CAD build for the part. Positions are in the model's coordinates, mm. Face numbers are marked on the shaded views. A direction names the side the tool comes from. Give positions to 0.01 mm unless a question says otherwise; leave off trailing zeros. Loops run counter-clockwise (first coordinate to the right, second up) from the corner with the lowest first, then second, coordinate; pieces in that order, holes last. Notation, with made-up numbers: (86, 31) -> (135, 31) arc R28 ccw to (135, 59) -> close; hole circle Ø3 at (79.25, 45.25). An arc over 180 degrees is marked (long way). Use one line per item in the form item = value.
```python
from build123d import *

# Parameters (mm, degrees)
F2_W     = 3
F2_H     = 3
F3_DEPTH = 9.201
F4_R     = 0.7
F5_DEPTH = 11.301


with BuildPart() as f1:
    # F0 (on Front) → F1 (revolve)
    with BuildSketch(Plane.XZ):
        Polygon((9.2, 8.05), (0, 8.05), (0.8, 6.6643593539), (0.8, 2.4), (9.4, 2.4), (10.3, 1.5), (14.8, 1.5), (14.8, 1.7), (27.8, 1.7), (27.8, 1.5), (33.8, 1.5), (33.8, 2.5), (33.2, 2.5), (33.2, 2.3), (32.5, 2.3), (32.5, 2.7), (12.1, 2.7), (12.1, 2.6), (11.3, 2.6), (11.3, 10), (9.2, 10), align=None)
    revolve(axis=Axis((16.7398190946, 0, 0), (1, 0, 0)))

    # F2 (on face) → F3 (cut, through all)
    with BuildSketch(Plane(origin=(9.2, 0, 0), x_dir=(0, -1, 0), z_dir=(-1, 0, 0))):
        with BuildLine():
            Line((1.5, 1.5), (1.5, 7.909013845))
            ThreePointArc((1.5, 7.909013845), (0, 8.05), (-1.5, 7.909013845))
            Line((-1.5, 7.909013845), (-1.5, 1.5))
            Line((-1.5, 1.5), (1.5, 1.5))
        make_face()
        with BuildLine():
            Line((1.5, 7.909013845), (1.5, 9.8868599666))
            ThreePointArc((1.5, 9.8868599666), (0, 10), (-1.5, 9.8868599666))
            Line((-1.5, 9.8868599666), (-1.5, 7.909013845))
            ThreePointArc((-1.5, 7.909013845), (0, 8.05), (1.5, 7.909013845))
        make_face()
        with BuildLine():
            Line((-1.5, -1.5), (-1.5, 1.5))
            Line((-1.5, 1.5), (-7.909013845, 1.5))
            ThreePointArc((-7.909013845, 1.5), (-8.05, 0), (-7.909013845, -1.5))
            Line((-7.909013845, -1.5), (-1.5, -1.5))
        make_face()
        with BuildLine():
            Line((-7.909013845, 1.5), (-9.8868599666, 1.5))
            ThreePointArc((-9.8868599666, 1.5), (-10, 0), (-9.8868599666, -1.5))
            Line((-9.8868599666, -1.5), (-7.909013845, -1.5))
            ThreePointArc((-7.909013845, -1.5), (-8.05, 0), (-7.909013845, 1.5))
        make_face()
        Rectangle(F2_W, F2_H)
        with BuildLine():
            ThreePointArc((8.05, 0), (8.0146759589, 0.7533055648), (7.909013845, 1.5))
            Line((7.909013845, 1.5), (1.5, 1.5))
            Line((1.5, 1.5), (1.5, -1.5))
            Line((1.5, -1.5), (7.909013845, -1.5))
            ThreePointArc((7.909013845, -1.5), (8.0146759589, -0.7533055648), (8.05, 0))
        make_face()
        with BuildLine():
            ThreePointArc((9.8868599666, -1.5), (9.971674876, -0.7521304187), (10, 0))
            ThreePointArc((10, 0), (9.971674876, 0.7521304187), (9.8868599666, 1.5))
            Line((9.8868599666, 1.5), (7.909013845, 1.5))
            ThreePointArc((7.909013845, 1.5), (8.0146759589, 0.7533055648), (8.05, 0))
            ThreePointArc((8.05, 0), (8.0146759589, -0.7533055648), (7.909013845, -1.5))
            Line((7.909013845, -1.5), (9.8868599666, -1.5))
        make_face()
        with BuildLine():
            ThreePointArc((-1.5, -7.909013845), (0, -8.05), (1.5, -7.909013845))
            Line((1.5, -7.909013845), (1.5, -1.5))
            Line((1.5, -1.5), (-1.5, -1.5))
            Line((-1.5, -1.5), (-1.5, -7.909013845))
        make_face()
        with BuildLine():
            ThreePointArc((-1.5, -9.8868599666), (0, -10), (1.5, -9.8868599666))
            Line((1.5, -9.8868599666), (1.5, -7.909013845))
            ThreePointArc((1.5, -7.909013845), (0, -8.05), (-1.5, -7.909013845))
            Line((-1.5, -7.909013845), (-1.5, -9.8868599666))
        make_face()
    extrude(amount=F3_DEPTH, mode=Mode.SUBTRACT)

    # F4 (on face) → F5 (cut, through all)
    with BuildSketch(Plane.YZ.offset(11.3)):
        with BuildLine():
            Line((-5.0204581464, 6.4346717088), (-6.3285168585, 7.7427304209))
            ThreePointArc((-6.3285168585, 7.7427304209), (-7.0710678119, 7.0710678119), (-7.7427304209, 6.3285168585))
            Line((-7.7427304209, 6.3285168585), (-6.4346717088, 5.0204581464))
            Line((-6.4346717088, 5.0204581464), (-5.0204581464, 6.4346717088))
        make_face()
        with Locations((0, 3.5)):
            Circle(F4_R)
        with Locations((0, -3.5)):
            Circle(F4_R)
    extrude(amount=-F5_DEPTH, mode=Mode.SUBTRACT)

    # F0 (on Front) → F6 (revolve, cut)
    with BuildSketch(Plane.XZ):
        Polygon((25.1366349399, -5.0709682839), (21.3, -0.0709682839), (21.3, -5.0709682839), align=None)
    revolve(axis=Axis((21.3, 0, -2.5709682839), (0, 0, -1)), mode=Mode.SUBTRACT)


solid = f1.part
```
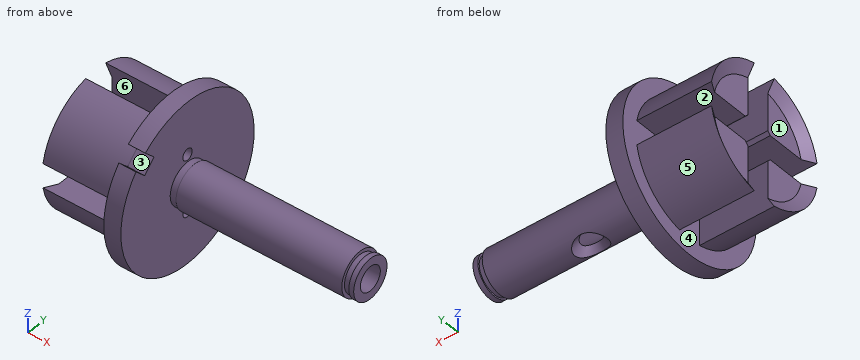
1. Mould opens along Z. For the marked faces 4, 5 and 6 say: pulls with the +Z half, pulls with the -Z half, needs draft (parallel to the pull), parting line crosses it, or undercut.
Result sheet:
face_4 = undercut
face_5 = pulls with the -Z half
face_6 = needs draft
2. Cut at C-C, the plane x = 31.5. Write the cut outline in (y, z).
Result sheet:
outline = circle Ø5.4 at (0, 0); hole circle Ø3 at (0, 0)
3. Cut at B-B, the plane y = 0. State how many separate pieces and enclosed holes the cut face has, then the cut area to 3 significant figures.
Result sheet:
separate_pieces = 5
enclosed_holes = 0
area = 73.2 mm^2
4. Drop flat-ended pins along their axis: P1, Ø2.5, axis at y = 0, z = -0.5, coming from the +X side; P2, Ø1.3, axis at y = 0, z = 3.5, coming from the +X side; P3, Ø4, axis at y = -3, z = 4, coming from the -X side; P4, Ø8, axis at x = 15.5, z = 5.5, coming from the +Y side (3 decimals). Give the stop position or say it passes through.
Result sheet:
P1 = 33.8
P2 = through
P3 = 0.61
P4 = 2.245
5. Drill centre lines: line 1 (Y direction, x = 23.5, z = 0); line 2 (Y direction, x = 14, z = 0). Where is each one in solid material? Low to high.
Result sheet:
line_1 = -2.7 to -1.7, 1.7 to 2.7
line_2 = -2.7 to -1.5, 1.5 to 2.7
6. Cut at A-A, the plane x = 18. Write the cut outline in (y, z).
Result sheet:
outline = circle Ø5.4 at (0, 0); hole circle Ø3.4 at (0, 0)
7. Tool access for the marked faces 1, 2 and 3: list every direction of +Z, -Z, +X, -X, +Y, -Y with a clear straight run to the whole face (end or side of a thin tool).
Result sheet:
face_1 = -X
face_2 = -X, +Y, -Y
face_3 = +X, -X
